Check sheet for the modelled part. Datum: model origin and axes. Units: mm. A direction names the side the tool comes from. Give positions to 0.01 mm unless a question says otherwise; leave off trailing zeros. Order: outer loops, then holes, each group sorted by start corner. A loop starts at its lowest first (then second) coordinate and runs counter-clockwise, first axis right, second up.
```python
from build123d import *

# Parameters (mm, degrees)
BOSS_EXTRUDE2_DEPTH = 6.35


with BuildPart() as part:
    # 3DSketch1 → Boss-Extrude2 (new body)
    with BuildSketch(Plane(origin=(4.175, -19.05, 0), x_dir=(-0.8568004384031221, 0.5156481443312075, 0), z_dir=(0, 0, -1))):
        with BuildLine():
            Line((0, 0), (9.168224006, 15.233911795))
            Line((9.168224006, 15.233911795), (-8.990144862, 26.162161584))
            ThreePointArc((-8.990144862, 26.162161584), (0.302776114, -7.593513786), (34.480876535, 0))
            Line((34.480876535, 0), (16.322507667, 10.92824979))
            Line((16.322507667, 10.92824979), (7.154283661, -4.305662005))
            Line((7.154283661, -4.305662005), (4.433942269, -2.668479147))
            Line((4.433942269, -2.668479147), (5.465238557, -0.95487827))
            Line((5.465238557, -0.95487827), (3.751637681, 0.076418019))
            Line((3.751637681, 0.076418019), (2.720341392, -1.637182858))
            Line((2.720341392, -1.637182858), (0, 0))
        make_face()
    extrude(amount=-BOSS_EXTRUDE2_DEPTH)


solid = part.part
```
(1) Cross-section at B-B on y = -10.5. Enter the section's corners in (x, z) (3 decimals).
Response values:
outline: (-23.128, 0) - (-4.175, 0) - (-4.175, 6.35) - (-23.128, 6.35) - close; (4.175, 0) - (23.128, 0) - (23.128, 6.35) - (4.175, 6.35) - close
(2) Release check for a two-part mould opening along X. For faces 3 (the face through (0.541, -25.394, 3.131)), 4 (the face through (-3, -19.05, 3)), 5 (the face through (15, -1.27, 3)) record: released by +X, released by -X, zero draft, split by the parting line, or undercut.
Response values:
face 3: split by the parting line
face 4: undercut
face 5: zero draft
(3) Cross-section at A-A on z = 4. Enter the section's corners in (x, y) (3 decimals), then the cut area to 3 significant figures.
Response values:
outline: (-25.368, -1.27) arc R25.4 ccw to (25.368, -1.27) - (4.175, -1.27) - (4.175, -19.05) - (1, -19.05) - (1, -17.05) - (-1, -17.05) - (-1, -19.05) - (-4.175, -19.05) - (-4.175, -1.27) - close
area: 804 mm2
(4) Cross-section at C-C on x = 0. Enter the section's corners in (y, z).
Response values:
outline: (-25.4, 0) - (-17.05, 0) - (-17.05, 6.35) - (-25.4, 6.35) - close
(5) Set-up check for faces 1 (the face through (-5, -14, 6.35)), 2 (the face through (1, -18, 3)): record each of +Z, -Z, +X, -X, +Y, -Y from which the full face is reachable in a straight line by a thin tool's end or side.
Response values:
face 1: +Z, +X, -X, +Y, -Y
face 2: +Z, -Z, +Y
(6) Gauge pin test, flat ends, axial feed: pin 1 Ø1.5 at (y, z) = (-22, 2) entering from -X; pin 2 Ø3.5 at (x, z) = (2, 3) entering from +Y; pin 3 Ø3 at (y, z) = (-18, 4.5) entering from +X. Record the tip position at first contact, or that the pin passes through.
Response values:
pin 1: stops at x = -13.91
pin 2: stops at y = -17.05
pin 3: stops at x = 19.31
(7) Cross-section at D-D on y = -15.75. Enter the section's corners in (x, z) (3 decimals), then the cut area to 3 significant figures.
Response values:
outline: (-19.927, 0) - (-4.175, 0) - (-4.175, 6.35) - (-19.927, 6.35) - close; (4.175, 0) - (19.927, 0) - (19.927, 6.35) - (4.175, 6.35) - close
area: 200 mm2
(8) Material ranges on L1, parallel to X at y = -14.5, z = 2 (1 decimal); L2, parallel to X at y = -3.75, z = 2 (3 decimals); L3, parallel to Y at x = 10, z = 4.5, recorded low to high.
Response values:
L1: x = -20.9 to -4.2, 4.2 to 20.9
L2: x = -25.122 to -4.175, 4.175 to 25.122
L3: y = -23.35 to -1.27
